Autodesk Inventor part; units mm, degrees
ref_plane "YZ Plane" through (0, 0, 0) normal (1, 0, 0) x (0, 1, 0)
ref_plane "XZ Plane" through (0, 0, 0) normal (0, 1, 0) x (-1, 0, 0)
ref_plane "XY Plane" through (0, 0, 0) normal (0, 0, 1) x (1, 0, 0)
sketch "Skizze1" plane through (0, 0, 0) normal (0, 0, 1) x (1, 0, 0)
  line L0 (4.0415, 0) -> (2.0207, -3.5)
  line L1 (2.0207, -3.5) -> (-2.0207, -3.5)
  line L2 (-2.0207, -3.5) -> (-4.0415, 0)
  line L3 (-4.0415, 0) -> (-2.0207, 3.5)
  line L4 (-2.0207, 3.5) -> (2.0207, 3.5)
  line L5 (2.0207, 3.5) -> (4.0415, 0)
  point P0 (0, 0)
  point P1 (0, 0)
  dimension "d0" = 7
extrude "Extrusion1" add sketch "Skizze1" along normal blind 20
sketch "Skizze2" plane through (0, 0, 20) normal (0, 0, 1) x (1, 0, 0)
  point P0 (0, 0)
hole "Bohrung1" at (0, 0, 20) direction (0, 0, -1) diameter 3.242 end through all
chamfer "Fase2" distance 0.7 angle 45 12 edges at (3.0311, -1.75, 20) (0, -3.5, 20) (-3.0311, -1.75, 20) (-3.0311, 1.75, 20) (0, 3.5, 20) (3.0311, 1.75, 20) (0, -3.5, 0) (3.0311, -1.75, 0) (3.0311, 1.75, 0) (0, 3.5, 0) (-3.0311, 1.75, 0) (-3.0311, -1.75, 0)
chamfer "Fase3" distance 0.2 angle 45 2 edges at (0, 1.621, 20) (0, 1.621, 0)
properties part number "Distanzhuelse_M4x20mm" material "Nickel-Kupfer-Legierung 400"
Here's how the part is built. I have some questions about the finished solid (model axes, mm). Round coordinates to 2 decimals unless told otherwise and drop trailing zeros. Write each loop counter-clockwise with the first axis right and the second up, starting at its lowest first coordinate (ties: lowest second). Pieces come first, ordered by that corner, then holes.
1. Will this pin go through, and if not, where does the flat tip stop? pin 1 Ø3 at (x, y) = (0, 0) entering from +Z.
2. Suppose I cut it at A-A (x = 0). List the corners of the cut face in (y, z) for me, and give its area (3 significant figures).
3. Suppose I cut it at C-C (y = -2.5). List the corners of the cut face in (x, z) for me, and give its area (3 significant figures).
4. Suppose I cut it at D-D (x = 3). List the corners of the cut face in (y, z) for me, and give its area (3 significant figures).
5. If we mould it in two halves opening along X, with no side actions, what happens to faces 1 (the cylindrical face through (1.438, -0.748, 9.863)), 2 (the flat face through (0, 2, 0)), 3 (the flat face through (-3.045, 1.726, 9.87))? For each: released by +X, released by -X, zero draft, split by the parting line, or undercut.
6. Suppose I cut it at B-B (z = 3.25). List the corners of the cut face in (x, y) for me.
7. I need wall thicknesses on L1, parallel to Y at x = 0, z = 14.75; L2, parallel to Y at x = -1.25, z = 19; L3, parallel to X at y = -0.25, z = 7. Which ranges of each line are inside material? Lowest first, please.
Answer sheet:
1. pin 1: passes through
2. outline: (-3.5, 0.7) - (-2.8, 0) - (-1.82, 0) - (-1.62, 0.2) - (-1.62, 19.8) - (-1.82, 20) - (-2.8, 20) - (-3.5, 19.3) - close; (1.62, 0.2) - (1.82, 0) - (2.8, 0) - (3.5, 0.7) - (3.5, 19.3) - (2.8, 20) - (1.82, 20) - (1.62, 19.8) - close
2. area: 74.1 mm2
3. outline: (-2.6, 0.7) - (-1.79, 0) - (1.79, 0) - (2.6, 0.7) - (2.6, 19.3) - (1.79, 20) - (-1.79, 20) - (-2.6, 19.3) - close
3. area: 103 mm2
4. outline: (-1.8, 0.7) - (-0.4, 0) - (0.4, 0) - (1.8, 0.7) - (1.8, 19.3) - (0.4, 20) - (-0.4, 20) - (-1.8, 19.3) - close
4. area: 70.2 mm2
5. face 1: undercut
5. face 2: zero draft
5. face 3: released by -X
6. outline: (-4.04, 0) - (-2.02, -3.5) - (2.02, -3.5) - (4.04, 0) - (2.02, 3.5) - (-2.02, 3.5) - close; hole circle Ø3.24 at (0, 0)
7. L1: y = -3.5 to -1.62, 1.62 to 3.5
7. L2: y = -3.5 to -1.03, 1.03 to 3.5
7. L3: x = -3.9 to -1.6, 1.6 to 3.9
